Print and shaded views of the part. All mm, measured from the part's lowest x, y and z. A direction names the side the tool comes from. Give positions to 0.01 mm unless a question says otherwise; leave off trailing zeros. Loops run counter-clockwise (first coordinate to the right, second up) from the corner with the lowest first, then second, coordinate; pieces in that order, holes last. Notation, with made-up numbers: (-14.5, 41.25) -> (13.5, 41.25) arc R27 ccw to (13.5, 75.25) -> close; hole circle Ø3 at (45, 1). An arc over 180 degrees is marked (long way). Write each question's results on one line, items separated by ' | '. Start each with the question number.
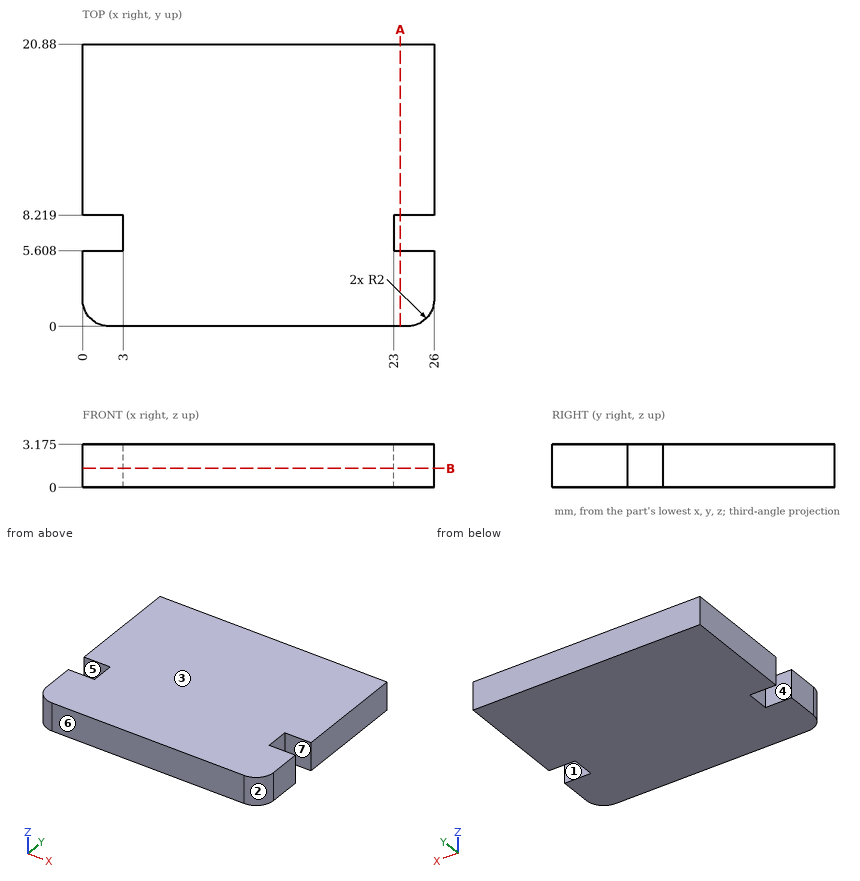
Q1. Drop flat-ended pins along their axis: pin 1 (1.5 mm diameter, centred on y = 7, z = 2, fed in from +X); pin 2 (0.9 mm diameter, centred on x = 1, z = 1.5, fed in from -Y). Give the stop position or say it passes through.
Q2. Saw through at B-B, the plane z = 1.4. List the corners of the cut face in (x, y).
Q3. Wall check: L1, parallel to Y at x = 2.25, z = 1.7; L2, parallel to X at y = 6.25, z = 2.25. Give the ranges that are in metal, low to high.
Q4. Saw through at A-A, the plane x = 23.5. List the corners of the cut face in (y, z) (1 decimal).
Q5. Which spindle directions (+Z, -Z, +X, -X, +Y, -Y) get a long thin tool onto all of the face, cutting with end or side? Do the marked faces 5, 6 and 7. Say none if no direction does.
Q6. Mould opens along Y. For the marked faces 1, 2, 3 and 4 say: pulls with the +Y half, pulls with the -Y half, needs draft (parallel to the pull), parting line crosses it, or undercut.
Answer block:
1) pin 1: stops at x = 23 | pin 2: stops at y = 0.08
2) outline: (0, 2) arc R2 ccw to (2, 0) -> (24, 0) arc R2 ccw to (26, 2) -> (26, 5.61) -> (23, 5.61) -> (23, 8.22) -> (26, 8.22) -> (26, 20.88) -> (0, 20.88) -> (0, 8.22) -> (3, 8.22) -> (3, 5.61) -> (0, 5.61) -> close
3) L1: y = 0 to 5.61, 8.22 to 20.88 | L2: x = 3 to 23
4) outline: (0, 0) -> (5.6, 0) -> (5.6, 3.2) -> (0, 3.2) -> close; (8.2, 0) -> (20.9, 0) -> (20.9, 3.2) -> (8.2, 3.2) -> close
5) face 5: +Z, -Z, -X | face 6: +Z, -Z, +X, -X, -Y | face 7: +Z, -Z, +X
6) face 1: undercut | face 2: pulls with the -Y half | face 3: needs draft | face 4: undercut
